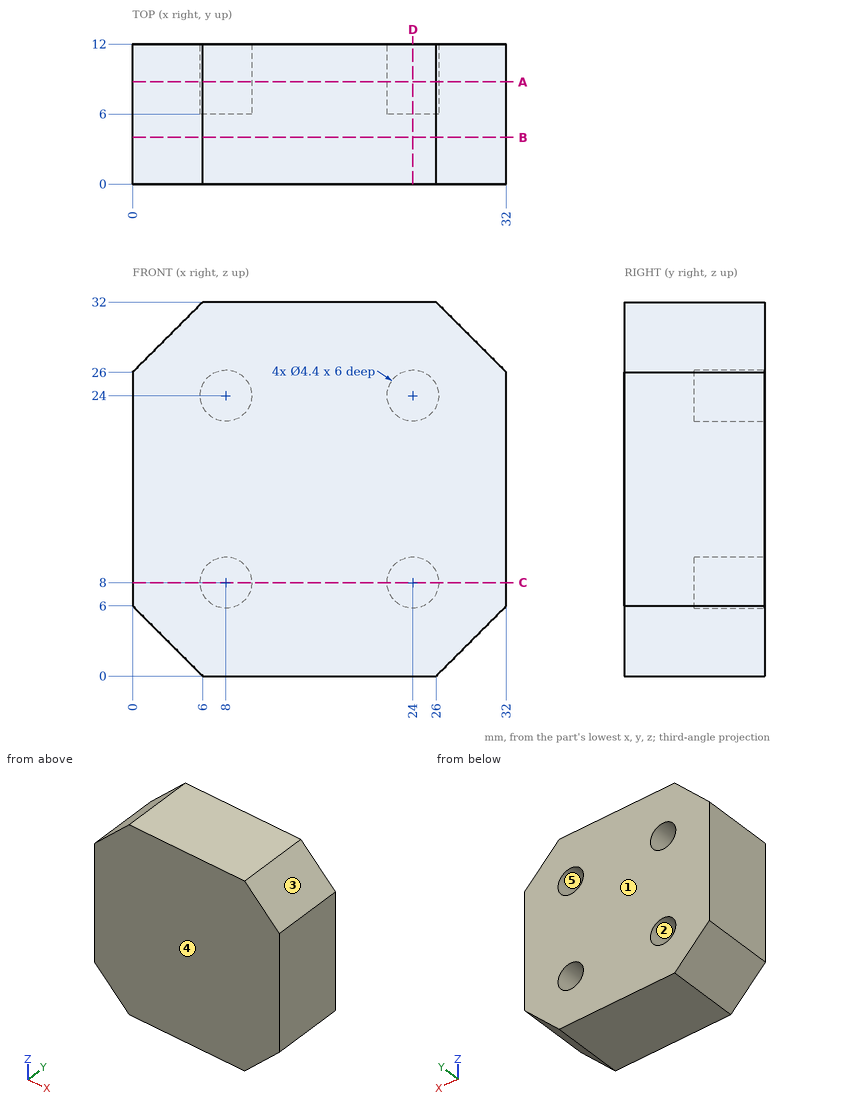
The figure shows three views and two pictorial views of one solid part (mm, origin at its lowest corner). Answer the questions. A direction names the side the tool comes from. Give positions to 0.01 mm unless a question says otherwise; leave off trailing zeros. Order: outer loops, then holes, each group sorted by start corner. A loop starts at its lowest first (then second) coordinate and runs counter-clockwise, first axis right, second up. Notation, with made-up numbers: M -36,79.25 L -13,79.25 A24 ccw -13,99.25 Z; hole C 15,-17.75 d7. An arc over 180 degrees is marked long. Return JSON: item names as keys, results as strings.
1) Straight lines are drawn through the part: line 1 along Z through (x, y) = (8, 9.05); line 2 along Z through (x, y) = (9, 11). For each, find the intervals that lie inside material, in ascending order. Write a range as [from, to].
Resolved:
{"line 1": "[0, 5.8], [10.2, 21.8], [26.2, 32]", "line 2": "[0, 6.04], [9.96, 22.04], [25.96, 32]"}
2) A tool of negligible diameter and unlimited length cuts with its end or side. For the marked faces 1 and 2, from which of +Z, -Z, +X, -X, +Y, -Y can it reach the whole face along a straight path? Write none if from no direction.
Resolved:
{"face 1": "+Z, -Z, +X, -X, +Y", "face 2": "+Y"}
3) Section A-A, the plane y = 8.75 is taken. Write down the section's boundary in (x, z).
Resolved:
{"outline": "M 0,6 L 6,0 L 26,0 L 32,6 L 32,26 L 26,32 L 6,32 L 0,26 Z; hole C 8,8 d4.4; hole C 8,24 d4.4; hole C 24,8 d4.4; hole C 24,24 d4.4"}
4) Section B-B, the plane y = 4 is taken. Write down the section's boundary in (x, z), plus the area to 3 significant figures.
Resolved:
{"outline": "M 0,6 L 6,0 L 26,0 L 32,6 L 32,26 L 26,32 L 6,32 L 0,26 Z", "area": "952 mm^2"}
5) This flat-tipped pin is pushed along its axis until it touches: pin 1 (4 mm diameter, centred on x = 24, z = 24, fed in from +Y). Where does it stop, or does it pass through?
Resolved:
{"pin 1": "y = 6"}
6) Section D-D, the plane x = 24 is taken. Write down the section's boundary in (y, z).
Resolved:
{"outline": "M 0,0 L 12,0 L 12,5.8 L 6,5.8 L 6,10.2 L 12,10.2 L 12,21.8 L 6,21.8 L 6,26.2 L 12,26.2 L 12,32 L 0,32 Z"}
7) For a pull along X with two mould halves and no side action, classify the marked faces 3, 4 and 5 as +X half, -X half, draft (parallel to the pull), parting line (faces both ways), or undercut.
Resolved:
{"face 3": "+X half", "face 4": "draft", "face 5": "undercut"}
8) Section C-C, the plane z = 8 is taken. Write down the section's boundary in (x, y).
Resolved:
{"outline": "M 0,0 L 32,0 L 32,12 L 26.2,12 L 26.2,6 L 21.8,6 L 21.8,12 L 10.2,12 L 10.2,6 L 5.8,6 L 5.8,12 L 0,12 Z"}
